from build123d import *

# Parameters (mm, degrees)
SKETCH1_W                       = 60
SKETCH1_H                       = 82.18
BOSS_EXTRUDE1_DEPTH             = 0.5
BOSS_EXTRUDE2_REACH             = 32
SKETCH3_R                       = 1
SKETCH3_R_2                     = 0.5
BOSS_EXTRUDE2_DIRECTION_2_REACH = 32
SKETCH4_R                       = 0.5
CUT_EXTRUDE1_DEPTH              = 61
SKETCH5_W                       = 48
SKETCH5_H                       = 1.968245837
SKETCH5_W_2                     = 1
CUT_EXTRUDE2_DEPTH              = 1.75
CUT_EXTRUDE2_DEPTH_BACK         = 2.25
BOSS_EXTRUDE3_DEPTH             = 1


with BuildPart() as part:
    # Sketch1 → Boss-Extrude1 (new body)
    with BuildSketch(Plane(origin=(0, 0, 0), x_dir=(1, 0, 0), z_dir=(0, 1, 0))):
        Rectangle(SKETCH1_W, SKETCH1_H)
    extrude(amount=BOSS_EXTRUDE1_DEPTH)

    # Boss-Extrude2: up to this face of the body (flat: up to its plane)
    boss_extrude2_end = Plane(part.part.faces().sort_by_distance((30, 0.25, 0))[0])
    # Sketch3 → Boss-Extrude2 (add, up to the picked face)
    with BuildSketch(Plane(origin=(0, 0, 0), x_dir=(0, 0, -1), z_dir=(1, 0, 0)), mode=Mode.PRIVATE) as boss_extrude2_sk1:
        with Locations((-41.09, 0.25)):
            Circle(SKETCH3_R)
        with Locations((-41.09, 0.25)):
            Circle(SKETCH3_R_2, mode=Mode.SUBTRACT)
    boss_extrude2_tool1 = split(extrude(boss_extrude2_sk1.sketch, amount=BOSS_EXTRUDE2_REACH, mode=Mode.PRIVATE), bisect_by=boss_extrude2_end, keep=Keep.BOTH, mode=Mode.PRIVATE)
    add(boss_extrude2_tool1.solids().sort_by_distance((0, 0.25, 42.061716))[0])

    # Boss-Extrude2 direction 2: up to this face of the body (flat: up to its plane)
    boss_extrude2_direction_2_end = Plane(part.part.faces().sort_by_distance((-30, 0.25, 0))[0])
    # Sketch3 → Boss-Extrude2 direction 2 (add, up to the picked face)
    with BuildSketch(Plane(origin=(0, 0, 0), x_dir=(0, 0, -1), z_dir=(1, 0, 0)), mode=Mode.PRIVATE) as boss_extrude2_direction_2_sk1:
        with Locations((-41.09, 0.25)):
            Circle(SKETCH3_R)
        with Locations((-41.09, 0.25)):
            Circle(SKETCH3_R_2, mode=Mode.SUBTRACT)
    boss_extrude2_direction_2_tool1 = split(extrude(boss_extrude2_direction_2_sk1.sketch, amount=-BOSS_EXTRUDE2_DIRECTION_2_REACH, mode=Mode.PRIVATE), bisect_by=boss_extrude2_direction_2_end, keep=Keep.BOTH, mode=Mode.PRIVATE)
    add(boss_extrude2_direction_2_tool1.solids().sort_by_distance((0, 0.25, 42.061716))[0])

    # Sketch4 → Cut-Extrude1 (cut, through all)
    with BuildSketch(Plane.ZY.offset(30)):
        with Locations((41.09, 0.25)):
            Circle(SKETCH4_R)
    extrude(amount=-CUT_EXTRUDE1_DEPTH, mode=Mode.SUBTRACT)

    # Sketch5 → Cut-Extrude2 (cut, two sides)
    with BuildSketch(Plane(origin=(0, 0.5, 0), x_dir=(1, 0, 0), z_dir=(0, 1, 0))) as cut_extrude2_sk:
        with Locations((0, -41.105877082)):
            Rectangle(SKETCH5_W, SKETCH5_H)
        with Locations((-29.5, -41.105877082)):
            Rectangle(SKETCH5_W_2, SKETCH5_H)
        with Locations((29.5, -41.105877082)):
            Rectangle(SKETCH5_W_2, SKETCH5_H)
    extrude(amount=CUT_EXTRUDE2_DEPTH, mode=Mode.SUBTRACT)
    extrude(cut_extrude2_sk.sketch, amount=-CUT_EXTRUDE2_DEPTH_BACK, mode=Mode.SUBTRACT)

    # Sketch7 → Boss-Extrude3 (add)
    with BuildSketch(Plane(origin=(0, 0, -41.09), x_dir=(-1, 0, 0), z_dir=(0, 0, -1))):
        with BuildLine():
            Line((-29, 0.5), (-28.25, 0.5))
            ThreePointArc((-28.25, 0.5), (-27.75, 1), (-27.25, 0.5))
            Line((-27.25, 0.5), (-26.5, 0.5))
            ThreePointArc((-26.5, 0.5), (-27.75, 1.75), (-29, 0.5))
        make_face()
    boss_extrude3 = extrude(amount=-BOSS_EXTRUDE3_DEPTH)

    # Mirror1: Boss-Extrude3 across plane
    add(boss_extrude3.mirror(Plane(origin=(0, 0, 0), x_dir=(0, 0, 1), z_dir=(1, 0, 0))))


solid = part.part
Geometry check sheet. Reference: the model listing, model coordinates, mm. A direction names the side the tool comes from. Round coordinates to 2 decimals unless told otherwise and drop trailing zeros. Order: outer loops, then holes, each group sorted by start corner. A loop starts at its lowest first (then second) coordinate and runs counter-clockwise, first axis right, second up. Notation, with made-up numbers: (-28, 88.5) -> (28, 88.5) arc R12 ccw to (28, 102.5) -> close; hole circle Ø1 at (4.25, 31.25). An arc over 180 degrees is marked (long way). Use one line per item in the form item = value.
1. Scan lines: line 1 along Z through (x, y) = (25.85, 0.25); line 2 along Y through (x, z) = (26.5, 41.09); line 3 along Y through (x, z) = (-23.5, -20). Record each from-to range of solid material in increasing order. Write a range as from..to.
Working result:
line_1 = -41.09..40.59, 41.59..42.09
line_2 = -0.75..-0.25, 0.75..1.25
line_3 = 0..0.5
2. Cross-section at A-A, the plane x = -15. Enter the section's corners in (y, z).
Working result:
outline = (0, -41.09) -> (0.5, -41.09) -> (0.5, 40.12) -> (0, 40.12) -> close
3. Cross-section at B-B, the plane z = 26.5. Enter the section's corners in (x, y).
Working result:
outline = (-30, 0) -> (30, 0) -> (30, 0.5) -> (-30, 0.5) -> close
4. Mould release check, pull along X, two halves, no side actions. Record for faces 4 (the face through (-24, 1, 41)), 5 (the face through (0, 0, -1)), 6 (the face through (-29, 1, 41)): pulls with the +X half, pulls with the -X half, needs draft (parallel to the pull), parting line crosses it, or undercut.
Working result:
face_4 = undercut
face_5 = needs draft
face_6 = pulls with the -X half
5. Go/stop test with flat-tipped pins: pin 1 (6 mm diameter, centred on x = -10, z = 9.5, fed in from +Y); pin 2 (0.6 mm diameter, centred on x = -28.5, y = 1, fed in from +Z); pin 3 (10 mm diameter, centred on x = 11.5, z = 31.5, fed in from -Y). Record where each tip stops, or that it passes through.
Working result:
pin_1 = 0.5
pin_2 = 41.98
pin_3 = 0
6. Set-up check for faces 1 (the face through (24, 1, 41)), 2 (the face through (29, 1, 41)), 3 (the face through (-7.1, 0.3, -41.09)): record each of +Z, -Z, +X, -X, +Y, -Y from which the full face is reachable in a straight line by a thin tool's end or side.
Working result:
face_1 = +Z, +Y, -Y
face_2 = +Z, +X, +Y, -Y
face_3 = -Z, +X, -X, +Y, -Y
